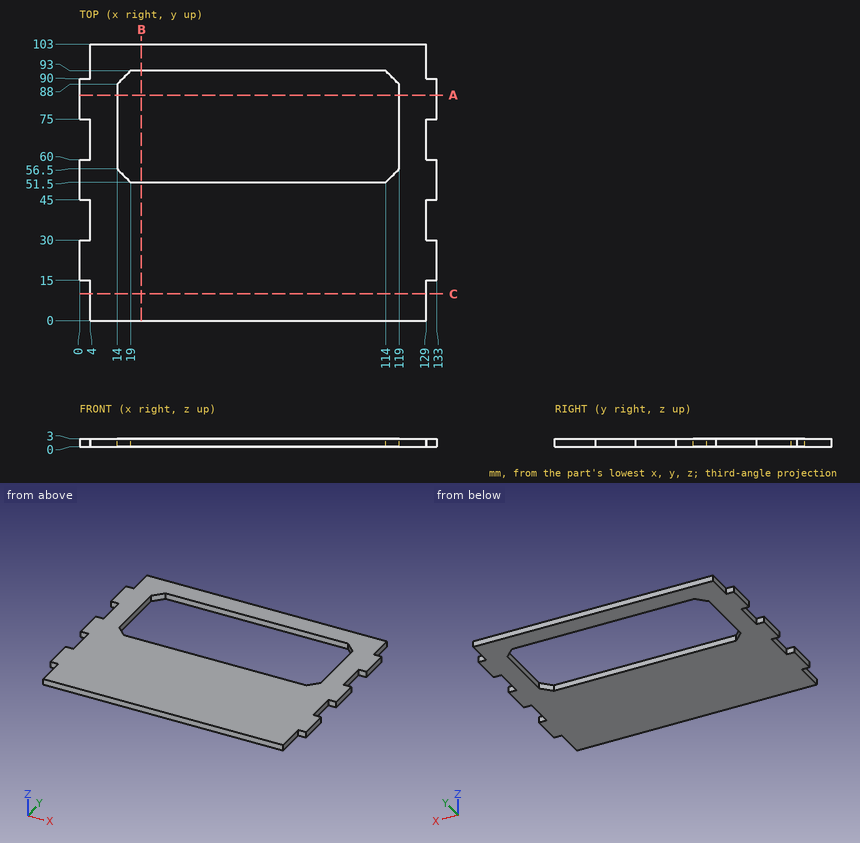
Answer from the drawing. Dimensions are ordinates in mm from the lowest x, y and z of the part. Round coordinates to 2 decimals unless told otherwise and drop trailing zeros. Write each loop counter-clockwise with the first axis right and the second up, starting at its lowest first coordinate (ties: lowest second). Pieces come first, ordered by that corner, then holes. Notation, with made-up numbers: (-36.75, 54.25) - (-5.75, 54.25) arc R26 cw to (-5.75, 89.25) - close; hole circle Ø5 at (23, -17). An arc over 180 degrees is marked (long way). One line per item, written item: value.
Q1. Find section A-A (y = 84). Determine the outline of the cut face in (x, z).
The answers:
outline: (0, 0) - (14, 0) - (14, 3) - (0, 3) - close; (119, 0) - (133, 0) - (133, 3) - (119, 3) - close
Q2. Straight lines are drawn through the part: line 1 (Y direction, x = 57.5, z = 1.15); line 2 (X direction, y = 59.5, z = 1); line 3 (X direction, y = 63, z = 0.1). For each, find the intervals that lie inside material, in ascending order. Write a range as from..to.
The answers:
line 1: y = 0..51.5, 93..103
line 2: x = 0..14, 119..133
line 3: x = 4..14, 119..129
Q3. Find section C-C (y = 10). Determine the outline of the cut face in (x, z).
The answers:
outline: (4, 0) - (129, 0) - (129, 3) - (4, 3) - close
Q4. Find section B-B (x = 23). Determine the outline of the cut face in (y, z), and give its area (4 significant figures).
The answers:
outline: (0, 0) - (51.5, 0) - (51.5, 3) - (0, 3) - close; (93, 0) - (103, 0) - (103, 3) - (93, 3) - close
area: 184.5 mm2
Q5. Each of these flat-tipped pins is pushed along its axis until it touches: P1, Ø0.9, axis at y = 70, z = 1, coming from the +X side; P2, Ø0.9, axis at x = 131.5, z = 1.5, coming from the -Y side; P3, Ø0.9, axis at y = 5.5, z = 1, coming from the -X side. Where does it stop, or does it pass through?
The answers:
P1: stops at x = 129
P2: stops at y = 15
P3: stops at x = 4
